CAD build for the part. Positions are in the model's coordinates, mm. A direction names the side the tool comes from. Round coordinates to 2 decimals unless told otherwise and drop trailing zeros. Loops run counter-clockwise (first coordinate to the right, second up) from the corner with the lowest first, then second, coordinate; pieces in that order, holes last. Notation, with made-up numbers: M 83,-14 L 88,-14 A29 cw 88,24 Z; hole C -34.5,-12.75 d3. An arc over 180 degrees is marked long. Put each result on its own line as item: value. Start each with the question number.
from build123d import *

# Parameters (mm, degrees)
SKETCH1_W           = 76.2
SKETCH1_H           = 30.48
BOSS_EXTRUDE1_DEPTH = 5.334
CAVITY1_START       = -171.988852232
CAVITY1_OUTLINE_W   = 30.48
CAVITY1_OUTLINE_H   = 5.334
CAVITY1_DEPTH       = 41.5925
SKETCH2_W           = 5.334
SKETCH2_H           = 6.35
BOSS_EXTRUDE2_DEPTH = 5.334
SKETCH3_W           = 13.788269566
SKETCH3_H           = 5.334
BOSS_EXTRUDE3_DEPTH = 5.334


# Read off the part's stored shape, not the designer's step: Cavity1
with BuildPart() as part:
    # Sketch1 → Boss-Extrude1 (new body)
    with BuildSketch(Plane.XY):
        with Locations((-133.888852232, -13.121247947)):
            Rectangle(SKETCH1_W, SKETCH1_H)
    extrude(amount=BOSS_EXTRUDE1_DEPTH)

    # Cavity1 outline → Cavity1 (cut)
    with BuildSketch(Plane.YZ.offset(CAVITY1_START)):
        with Locations((-13.121247947, 2.667)):
            Rectangle(CAVITY1_OUTLINE_W, CAVITY1_OUTLINE_H)
    extrude(amount=CAVITY1_DEPTH, mode=Mode.SUBTRACT)

    # Sketch2 → Boss-Extrude2 (add)
    with BuildSketch(Plane.XY.offset(5.334)):
        with Locations((-133.063352232, -19.80374181)):
            Rectangle(SKETCH2_W, SKETCH2_H)
    extrude(amount=-BOSS_EXTRUDE2_DEPTH)

    # Sketch3 → Boss-Extrude3 (add)
    with BuildSketch(Plane.XY.offset(5.334)):
        with Locations((-113.775970546, -31.028247947)):
            Rectangle(SKETCH3_W, SKETCH3_H)
    extrude(amount=-BOSS_EXTRUDE3_DEPTH)


solid = part.part
(1) Tool access for faces 1 (the flat face through (-133, -16.629, 3)), 2 (the flat face through (-116, -16, 0)), 3 (the flat face through (-130.396, -26, 3)), 4 (the flat face through (-101, -28.361, 3)): list every direction of +Z, -Z, +X, -X, +Y, -Y with a clear straight run to the whole face (end or side of a thin tool).
(2) Flat gauge pins, fed straight in: pin 1 Ø2.5 at (x, z) = (-103, 2) entering from -Y; pin 2 Ø2.5 at (y, z) = (-24.5, 3.5) entering from -X; pin 3 Ø2.5 at (x, z) = (-133.5, 2) entering from -Y. Where does each tip first touch, or does it go through?
(3) Drill centre lines: line 1 along Y through (x, z) = (-128, 0.3); line 2 along X through (y, z) = (-30.5, 1.7); line 3 along X through (y, z) = (-3.5, 3.75). Where is each one in solid material? Low to high.
(4) Cut at B-B on x = -123. List the corners of the cut face in (y, z), and give its area (3 significant figures).
(5) Cut at C-C on y = -27.5. List the corners of the cut face in (x, z), and give its area (3 significant figures).
(6) Cut at A-A on z = 4.25. List the corners of the cut face in (x, y), and give its area (3 significant figures).
Taken from the geometry:
1. face 1: +Z, -Z, -X, +Y
1. face 2: -Z, +X, -X, +Y, -Y
1. face 3: +Z, -Z, -X, -Y
1. face 4: +Z, -Z, +X, -Y
2. pin 1: y = -28.36
2. pin 2: x = -130.4
2. pin 3: y = -22.98
3. line 1: -28.36 to 2.12
3. line 2: -120.67 to -106.88
3. line 3: -130.4 to -95.79
4. outline: M -28.36,0 L 2.12,0 L 2.12,5.33 L -28.36,5.33 Z
4. area: 163 mm2
5. outline: M -130.4,0 L -95.79,0 L -95.79,5.33 L -130.4,5.33 Z
5. area: 185 mm2
6. outline: M -135.73,-22.98 L -130.4,-22.98 L -130.4,-28.36 L -120.67,-28.36 L -120.67,-33.7 L -106.88,-33.7 L -106.88,-28.36 L -95.79,-28.36 L -95.79,2.12 L -130.4,2.12 L -130.4,-16.63 L -135.73,-16.63 Z
6. area: 1,160 mm2
